from build123d import *

# Parameters (mm, degrees)
F0_R     = 10
F1_DEPTH = 25
F3_ANGLE = -45
F5_ANGLE = -45


with BuildPart() as f1:
    # F0 (on Top) → F1 (new body)
    with BuildSketch(Plane.XY):
        Circle(F0_R)
    extrude(amount=F1_DEPTH)

    # F2 (on Front) → F3 (revolve, cut)
    with BuildSketch(Plane.XZ):
        with BuildLine():
            Line((11, 12), (11, 15))
            ThreePointArc((11, 15), (9.5, 13.5), (11, 12))
        make_face()
    revolve(axis=Axis((0, 0, 25), (0, 0, 1)), revolution_arc=F3_ANGLE, mode=Mode.SUBTRACT)


with BuildPart() as f4:
    # F2 (on Front) → F4 (revolve)
    with BuildSketch(Plane.XZ):
        with BuildLine():
            Line((11, 12), (11, 15))
            ThreePointArc((11, 15), (9.5, 13.5), (11, 12))
        make_face()
    revolve(axis=Axis((11, 0, 13.5), (0, 0, -1)))


with BuildPart() as f5_1:
    # F5: copy of F4
    add(f4.part.rotate(Axis((0, 0, 25), (0, 0, 1)), F5_ANGLE))


with BuildPart() as f1_1:
    add(f1.part)

    # F6: cut F5_1, F4
    add(f5_1.part, mode=Mode.SUBTRACT)
    add(f4.part, mode=Mode.SUBTRACT)


solid = f1_1.part
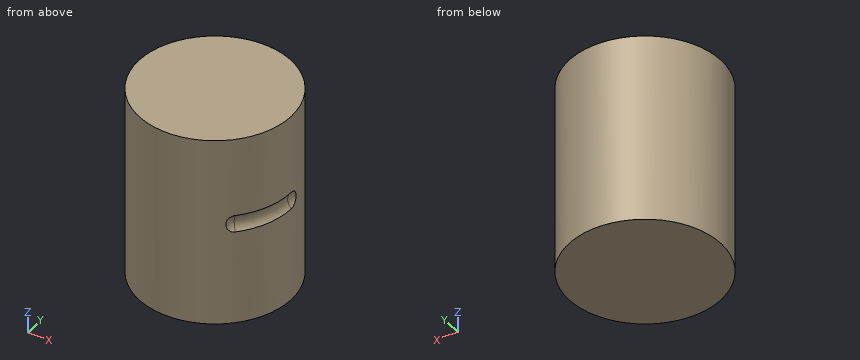
Model file for the job. Use its own axes, mm. Give positions to 0.01 mm unless a question says otherwise; leave off trailing zeros. Order: outer loops, then holes, each group sorted by start corner. A loop starts at its lowest first (then second) coordinate and runs counter-clockwise, first axis right, second up. Notation, with made-up numbers: (7, 22.5) -> (61, 22.5) arc R19 ccw to (61, 28.5) -> close; hole circle Ø11 at (1, 22). An arc over 180 degrees is marked (long way). Use CSV: the item, a comma, the result in double quotes.
1. Band-saw the part on A-A, the plane z = 8. Give the cut face in (x, y).
Outcome:
outline,"circle Ø20 at (0, 0)"
2. Band-saw the part on B-B, the plane x = 3.25. Give the cut face in (y, z), then the cut area to 3 significant figures.
Outcome:
outline,"(-9.46, 0) -> (9.46, 0) -> (9.46, 25) -> (-9.46, 25) -> close"
area,"473 mm²"
3. Drill centre lines: line 1 along X through (y, z) = (6.25, 23.75); line 2 along X through (y, z) = (-3.5, 1.25); line 3 along Y through (x, z) = (-6, 15.75). Where is each one in solid material? Low to high. Write a range as from..to.
Outcome:
line 1,"-7.81..7.81"
line 2,"-9.37..9.37"
line 3,"-8..8"
4. Drop flat-ended pins along their axis: pin 1 (12 mm diameter, centred on x = -7.5, z = 12.5, fed in from -Y); pin 2 (12 mm diameter, centred on y = -4, z = 4.5, fed in from +X); pin 3 (1.5 mm diameter, centred on y = 7.5, z = 20, fed in from -X); pin 4 (6 mm diameter, centred on x = -7, z = 19.5, fed in from -Y). Give the stop position or say it passes through.
Outcome:
pin 1,"y = -9.89"
pin 2,"x = 10"
pin 3,"x = -7.38"
pin 4,"y = -9.17"
5. Band-saw the part on C-C, the plane y = 1.75. Give the cut face in (x, z).
Outcome:
outline,"(-9.85, 0) -> (9.85, 0) -> (9.85, 25) -> (-9.85, 25) -> close"
